The model under review builds one solid part; all positions refer to its coordinate system, in mm. A direction names the side the tool comes from. Round coordinates to 2 decimals unless told otherwise and drop trailing zeros. Order: outer loops, then holes, each group sorted by start corner. A loop starts at its lowest first (then second) coordinate and runs counter-clockwise, first axis right, second up.
1) Consider section C-C (y = 1.75). Give the boundary of the cut face in (x, z).
2) Consider section B-B (x = 0). Give the boundary of the cut face in (y, z).
3) Clearance check with flat-ended pins moving along their axes: P1, Ø6, axis at x = -9, y = 18.5, coming from the -Z side; P2, Ø5, axis at x = 6, z = -0.5, coming from the -Y side; P3, Ø5, axis at x = -3.5, z = -2, coming from the -Y side. State where each tip first meets the part, or that it passes through.
4) Machinability: for faces 4 (the face through (-1.64, 15.954, 7.386)), 5 (the face through (0, 10, 0)), which of the approach directions +Z, -Z, +X, -X, +Y, -Y give a long, thin tool a straight path to every point of the face, cutting with its end or side? Answer none if there is none.
5) To check wall thickness, follow L1, parallel to Y at x = 0.25, z = 1; L2, parallel to Y at x = -2.5, z = 9.25; L3, parallel to X at y = 3.25, z = -0.5. State the ranges of each line that lie inside material, in increasing order.
6) Consider section A-A (z = 0). Give the boundary of the cut face in (x, y), then the cut area to 3 significant figures.
7) Mouldability with a two-part tool opening along X and no side actions: class faces 1 (the face through (-3, 5, 0)), 2 (the face through (0, 22, 0)), 3 (the face through (11.923, 1.549, -3.755)) as pulls with the +X half, pulls with the -X half, needs draft (parallel to the pull), parting line crosses it, or undercut.
8) Consider section D-D (y = 14.25). Give the boundary of the cut face in (x, z).
from build123d import *

# Parameters (mm, degrees)
SKETCH3_R          = 3
CUT_EXTRUDE1_DEPTH = 10


with BuildPart() as part:
    # Sketch2 → Revolve1 (revolve)
    with BuildSketch(Plane.XY):
        Polygon((0, 0), (5, 0), (10.5, -2), (12.5, -2), (12.5, 5), (9.291654184, 6.167742378), (6.5, 22), (0, 22), align=None)
    revolve(axis=Axis((0, -4.501967694, 0), (0, 1, 0)))

    # Sketch3 → Cut-Extrude1 (cut)
    with BuildSketch(Plane.XZ):
        Circle(SKETCH3_R)
    extrude(amount=-CUT_EXTRUDE1_DEPTH, mode=Mode.SUBTRACT)


solid = part.part
Answer below:
1. outline: circle Ø25 at (0, 0); hole circle Ø6 at (0, 0)
2. outline: (-2, -12.5) - (5, -12.5) - (6.17, -9.29) - (22, -6.5) - (22, 6.5) - (6.17, 9.29) - (5, 12.5) - (-2, 12.5) - (-2, 10.5) - (0, 5) - (0, 3) - (10, 3) - (10, -3) - (0, -3) - (0, -5) - (-2, -10.5) - close
3. P1: stops at z = -3.93
3. P2: stops at y = -1.28
3. P3: stops at y = -0.56
4. face 4: +Y
4. face 5: -Y
5. L1: y = 10 to 22
5. L2: y = -1.67 to 6.06
5. L3: x = -12.49 to -2.96, 2.96 to 12.49
6. outline: (-12.5, -2) - (-10.5, -2) - (-5, 0) - (-3, 0) - (-3, 10) - (3, 10) - (3, 0) - (5, 0) - (10.5, -2) - (12.5, -2) - (12.5, 5) - (9.29, 6.17) - (6.5, 22) - (-6.5, 22) - (-9.29, 6.17) - (-12.5, 5) - close
6. area: 359 mm2
7. face 1: undercut
7. face 2: needs draft
7. face 3: parting line crosses it
8. outline: circle Ø15.73 at (0, 0)
